Source: CAD feature listing. Evaluate the final solid. Frame: model axes, mm. Round coordinates to 2 decimals unless told otherwise and drop trailing zeros. Write each loop counter-clockwise with the first axis right and the second up, starting at its lowest first coordinate (ties: lowest second). Pieces come first, ordered by that corner, then holes. Notation, with made-up numbers: (66.25, -14) - (110.25, -14) arc R21 cw to (110.25, -5) - close; hole circle Ø4 at (34.25, 33). An arc over 180 degrees is marked (long way). Write item = value, one per line. Start each with the question number.
Autodesk Inventor part; units mm, degrees
ref_plane "YZ Plane" through (0, 0, 0) normal (1, 0, 0) x (0, 1, 0)
ref_plane "XZ Plane" through (0, 0, 0) normal (0, 1, 0) x (-1, 0, 0)
ref_plane "XY Plane" through (0, 0, 0) normal (0, 0, 1) x (1, 0, 0)
sketch "Sketch1" plane through (0, 0, 0) normal (0, 1, 0) x (-1, 0, 0)
  line L0 (-139.7, 292.1) -> (139.7, 292.1)
  line L1 (139.7, 292.1) -> (139.7, -292.1)
  line L2 (139.7, -292.1) -> (-139.7, -292.1)
  line L3 (-139.7, -292.1) -> (-139.7, -89.789)
  line L4 (-139.7, 292.1) -> (139.7, -292.1) construction
  line L5 (139.7, 292.1) -> (-139.7, -292.1) construction
  line L6 (-152.4, 304.8) -> (152.4, 304.8)
  line L7 (152.4, 304.8) -> (152.4, -304.8)
  line L8 (152.4, -304.8) -> (-152.4, -304.8)
  line L9 (-152.4, -304.8) -> (-152.4, -89.789)
  line L10 (-152.4, 304.8) -> (152.4, -304.8) construction
  line L11 (152.4, 304.8) -> (-152.4, -304.8) construction
  line L12 (40.5945, 180.2806) -> (144.9885, 180.2806)
  line L13 (144.9885, 180.2806) -> (144.9885, -1.9898)
  line L14 (144.9885, -1.9898) -> (40.5945, -1.9898)
  line L15 (40.5945, -1.9898) -> (40.5945, 180.2806)
  line L16 (40.5945, 180.2806) -> (144.9885, -1.9898) construction
  line L17 (144.9885, 180.2806) -> (40.5945, -1.9898) construction
  line L18 (145.8849, -184.8763) -> (19.2151, -184.8763)
  line L19 (19.2151, -184.8763) -> (19.2151, -55.4887)
  line L20 (19.2151, -55.4887) -> (145.8849, -55.4887)
  line L21 (145.8849, -55.4887) -> (145.8849, -184.8763)
  line L22 (145.8849, -184.8763) -> (19.2151, -55.4887) construction
  line L23 (19.2151, -184.8763) -> (145.8849, -55.4887) construction
  line L24 (122.3815, 273.05) -> (73.9219, 273.05)
  line L25 (73.9219, 273.05) -> (73.9219, 209.9282)
  line L26 (73.9219, 209.9282) -> (122.3815, 209.9282)
  line L27 (122.3815, 209.9282) -> (122.3815, 273.05)
  line L28 (122.3815, 273.05) -> (73.9219, 209.9282) construction
  line L29 (54.8719, 273.05) -> (6.4122, 273.05)
  line L30 (6.4122, 273.05) -> (6.4122, 209.9282)
  line L31 (6.4122, 209.9282) -> (54.8719, 209.9282)
  line L32 (54.8719, 209.9282) -> (54.8719, 273.05)
  line L33 (-12.6378, 273.05) -> (-61.0974, 273.05)
  line L34 (-61.0974, 273.05) -> (-61.0974, 209.9282)
  line L35 (-61.0974, 209.9282) -> (-12.6378, 209.9282)
  line L36 (-12.6378, 209.9282) -> (-12.6378, 273.05)
  line L37 (-80.1474, 273.05) -> (-128.607, 273.05)
  line L38 (-128.607, 273.05) -> (-128.607, 209.9282)
  line L39 (-128.607, 209.9282) -> (-80.1474, 209.9282)
  line L40 (-80.1474, 209.9282) -> (-80.1474, 273.05)
  line L41 (73.9219, 273.05) -> (122.3815, 209.9282)
  line L42 (6.4122, 273.05) -> (54.8719, 209.9282)
  line L43 (-61.0974, 273.05) -> (-12.6378, 209.9282)
  line L44 (-128.607, 273.05) -> (-80.1474, 209.9282)
  line L45 (139.7, -18.3929) -> (25.4, -18.3929)
  line L46 (25.4, -18.3929) -> (25.4, -208.8929)
  line L47 (25.4, -208.8929) -> (139.7, -208.8929)
  line L48 (139.7, -208.8929) -> (139.7, -18.3929)
  line L49 (-44.45, -89.789) -> (-152.4, -89.789)
  line L50 (-44.45, 89.789) -> (-44.45, -89.789)
  line L51 (-152.4, 89.789) -> (-44.45, 89.789)
  line L52 (-139.7, 89.789) -> (-139.7, 292.1)
  line L53 (-152.4, 89.789) -> (-152.4, 304.8)
  point P0 (0, 0)
  point P1 (0, 0)
  point P2 (0, 0)
  point P3 (92.7915, 89.1454)
  point P4 (92.7915, 89.1454)
  point P5 (82.55, -120.1825)
  point P6 (82.55, -120.1825)
  point P7 (108.7202, 255.2553)
  point P8 (82.55, -120.1825)
  point P9 (-152.4, 0)
  dimension "d71" = 279.4
  dimension "d72" = 584.2
  dimension "d73" = 304.8
  dimension "d74" = 609.6
  dimension "d84" = 104.394
  dimension "d85" = 182.2704
  dimension "d86" = 126.6698
  dimension "d87" = 129.3876
  dimension "d102" = 19.05
  dimension "d103" = 19.05
  dimension "d104" = 19.05
  dimension "d112" = 79.5782
  dimension "d113" = 79.5782
  dimension "d114" = 79.5782
  dimension "d115" = 79.5782
  dimension "d116" = 114.3
  dimension "d117" = 190.5
  dimension "d127" = 179.578
  dimension "d128" = 107.95
  dimension "d129" = 107.95
  dimension "d130" = 52.486
  dimension "d134" = 298.6819
  dimension "d135" = 30.0185
  dimension "d137" = 12.7
  dimension "d138" = 31.75
extrude "Extrusion6" add sketch "Sketch1" along normal blind 6.35 contours L52 L51 L53 L6 L7 L8 L9 L49 L3 L2 L1 L18 L21 L20 L14 L13 L12 L0 | L0 L1 L12 L15 L14 L45 L46 L20 L19 L18 L47 L2 L3 L49 L50 L51 L52 | L12 L13 L14 L1 | L1 L14 L15 L12 | L1 L20 L46 L45 | L20 L21 L18 L1 | L1 L18 L46 L20 | L1 L47 L46 L18 | L46 L18 L19 L20 | L27 L41 L24 | L41 L26 L25 | L32 L42 L29 | L42 L31 L30 | L36 L43 L33 | L43 L35 L34 | L40 L44 L37 | L44 L39 L38
hole "Hole6" at (139.7, 0, 292.1) at (-139.7, 0, 292.1) at (-139.7, 0, -292.1) at (139.7, 0, -292.1) at (-19.2151, 0, -55.4887) at (-19.2151, 0, -184.8763) at (-145.8849, 0, -184.8763) at (-145.8849, 0, -55.4887) at (-144.9885, 0, 180.2806) at (-40.5945, 0, 180.2806) at (-40.5945, 0, -1.9898) at (-144.9885, 0, -1.9898) direction (0, 1, 0) diameter 6.35 end through all
hole "Hole7" at (-122.3815, 0, 209.9282) at (-73.9219, 0, 273.05) at (-54.8719, 0, 209.9282) at (-6.4122, 0, 273.05) at (12.6378, 0, 209.9282) at (61.0974, 0, 273.05) at (80.1474, 0, 209.9282) at (128.607, 0, 273.05) direction (0, 1, 0) diameter 3.81 end through all
hole "Hole8" at (-139.7, 0, -18.3929) at (-25.4, 0, -18.3929) at (-25.4, 0, -208.8929) at (-139.7, 0, -208.8929) direction (0, 1, 0) diameter 6.35 end through all
properties part number "eboardbaseplate"
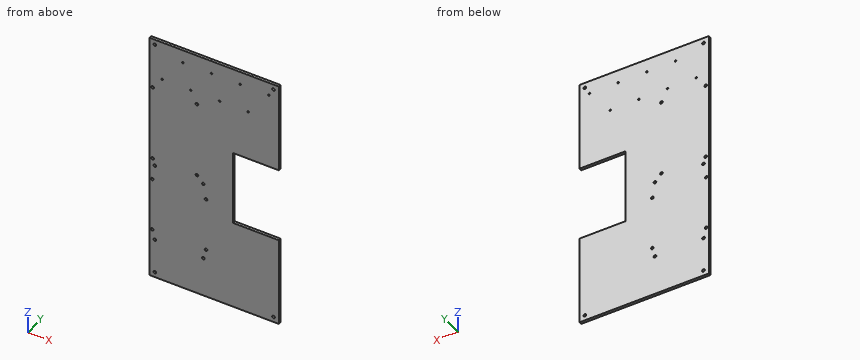
(1) Section B-B (z = 30.5). Return the cut outline in (x, y), plus the area to 3 significant figures.
(2) Section A-A (y = 3). Count the separate pieces of the cut face and the enclosed holes in it, plus the area to 3 significant figures.
(3) Contact query for flat-ended pins moving along their axis: P1, Ø4, axis at x = -25.4, z = -18.39, coming from the -Y side; P2, Ø3, axis at y = 3, z = -27.5, coming from the +X side; P3, Ø8.5, axis at x = -144.99, z = 180.28, coming from the +Y side. Output: stop coordinate, or through.
(4) Ray query, L1, parallel to X at y = 3.5, z = -184.5; L2, parallel to Z at x = 91.5, y = 6; L3, parallel to Z at x = 139.7, y = 5.25 (3 decimals). Return the intervals inside material, ascending. Write a range as from..to.
Solution:
q1.outline = (-152.4, 0) - (44.45, 0) - (44.45, 6.35) - (-152.4, 6.35) - close
q1.area = 1,250 mm^2
q2.separate_pieces = 1
q2.enclosed_holes = 24
q2.area = 166,000 mm^2
q3.P1 = through
q3.P2 = 44.45
q3.P3 = 6.35
q4.L1 = -152.4..-149.04, -142.73..-22.37, -16.06..152.4
q4.L2 = -304.8..-89.79, 89.79..304.8
q4.L3 = -304.8..-295.275, -288.925..-89.789, 89.789..288.925, 295.275..304.8
